Model file for the job. Use its own axes, mm. A direction names the side the tool comes from. Give positions to 0.01 mm unless a question says otherwise; leave off trailing zeros. Loops run counter-clockwise (first coordinate to the right, second up) from the corner with the lowest first, then second, coordinate; pieces in that order, holes last. Notation, with made-up numbers: M 70,2.5 L 86,2.5 A26 cw 86,25.5 Z; hole C -34,65 d11. An arc over 180 degrees is marked long. Answer in a Markdown table with one row per item.
```python
from build123d import *

# Parameters (mm, degrees)
STOCK_ECCENTRIC_START               = 21
STOCK_ECCENTRIC_SHAFT_1_OUTLINE_R   = 10
STOCK_ECCENTRIC_SHAFT_1_OUTLINE_R_2 = 1.5
STOCK_ECCENTRIC_SHAFT_1_DEPTH       = 9
STOCK_ECCENTRIC_START_2             = 30
STOCK_ECCENTRIC_SHAFT_1_2_DEPTH     = 1
BOSS_EXTRUDE1_START                 = 1
SKETCH1_R                           = 10
SKETCH1_R_2                         = 1.5
BOSS_EXTRUDE1_DEPTH                 = 1
CUT_EXTRUDE1_START                  = -1
CUT_EXTRUDE1_DEPTH                  = 1


# Read off the part's stored shape, not the designer's step: Stock-Eccentric Shaft-1
with BuildPart() as part:
    # Stock-Eccentric Shaft-1 outline → Stock-Eccentric Shaft-1 (new body)
    with BuildSketch(Plane(origin=(0, 0, 0), x_dir=(1, 0, 0), z_dir=(0, 1, 0)).offset(STOCK_ECCENTRIC_START)):
        with Locations((-2.5, 0)):
            Circle(STOCK_ECCENTRIC_SHAFT_1_OUTLINE_R)
        with Locations((-4, 0)):
            Circle(STOCK_ECCENTRIC_SHAFT_1_OUTLINE_R_2, mode=Mode.SUBTRACT)
        with Locations((4, 0)):
            Circle(STOCK_ECCENTRIC_SHAFT_1_OUTLINE_R_2, mode=Mode.SUBTRACT)
    extrude(amount=STOCK_ECCENTRIC_SHAFT_1_DEPTH)

    # Stock-Eccentric Shaft-1 2 outline → Stock-Eccentric Shaft-1 2 (add)
    with BuildSketch(Plane(origin=(0, 0, 0), x_dir=(1, 0, 0), z_dir=(0, 1, 0)).offset(STOCK_ECCENTRIC_START_2)):
        with BuildLine():
            ThreePointArc((-10.712142643, 2.5), (-8.817418729, 6.576710953), (-5.45, 9.554972527))
            ThreePointArc((-5.45, 9.554972527), (-9.734494483, 6.903773575), (-12.182458366, 2.5))
            Line((-12.182458366, 2.5), (-10.712142643, 2.5))
        make_face()
        with BuildLine():
            ThreePointArc((-12.182458366, -2.5), (-9.734494483, -6.903773575), (-5.45, -9.554972527))
            ThreePointArc((-5.45, -9.554972527), (-8.817418729, -6.576710953), (-10.712142643, -2.5))
            Line((-10.712142643, -2.5), (-12.182458366, -2.5))
        make_face()
    extrude(amount=STOCK_ECCENTRIC_SHAFT_1_2_DEPTH)

    # Sketch1 → Boss-Extrude1 (add)
    # profile 1 of 4: a face of its own
    with BuildSketch(Plane.XZ.offset(-21).offset(BOSS_EXTRUDE1_START)):
        with BuildLine():
            Line((7.928326807, -3.5), (7.8, -3.5))
            Line((7.8, -3.5), (7.8, 3.5))
            Line((7.8, 3.5), (7.928326807, 3.5))
            ThreePointArc((7.928326807, 3.5), (-13.5, 0), (7.928326807, -3.5))
        make_face()
        with Locations(Location((-2.5, 0, 0), (0, 0, 252.842462628))):
            Circle(SKETCH1_R, mode=Mode.SUBTRACT)
    # profile 2 of 4: a face of its own
    with BuildSketch(Plane.XZ.offset(-21).offset(BOSS_EXTRUDE1_START)):
        with Locations(Location((-2.5, 0, 0), (0, 0, 252.842462628))):
            Circle(SKETCH1_R)
        with Locations(Location((4, 0, 0), (0, 0, 90))):
            Circle(SKETCH1_R_2, mode=Mode.SUBTRACT)
        with Locations(Location((-4, 0, 0), (0, 0, 90))):
            Circle(SKETCH1_R_2, mode=Mode.SUBTRACT)
    # profile 3 of 4: a face of its own
    with BuildSketch(Plane.XZ.offset(-21).offset(BOSS_EXTRUDE1_START)):
        with BuildLine():
            Line((7.8, 3.5), (7.8, -3.5))
            Line((7.8, -3.5), (7.928326807, -3.5))
            ThreePointArc((7.928326807, -3.5), (8.356141001, -1.773189939), (8.5, 0))
            ThreePointArc((8.5, 0), (8.356141001, 1.773189939), (7.928326807, 3.5))
            Line((7.928326807, 3.5), (7.8, 3.5))
        make_face()
    # profile 4 of 4: a face of its own
    with BuildSketch(Plane.XZ.offset(-21).offset(BOSS_EXTRUDE1_START)):
        with BuildLine():
            ThreePointArc((8.5, 0), (8.356141001, -1.773189939), (7.928326807, -3.5))
            Line((7.928326807, -3.5), (10.8, -3.5))
            Line((10.8, -3.5), (10.8, 3.5))
            Line((10.8, 3.5), (7.928326807, 3.5))
            ThreePointArc((7.928326807, 3.5), (8.356141001, 1.773189939), (8.5, 0))
        make_face()
    extrude(amount=-BOSS_EXTRUDE1_DEPTH)

    # Sketch2 → Cut-Extrude1 (cut)
    with BuildSketch(Plane(origin=(0, 31, 0), x_dir=(1, 0, 0), z_dir=(0, 1, 0)).offset(CUT_EXTRUDE1_START)):
        with BuildLine():
            ThreePointArc((-5.45, 9.554972527), (-6.473664245, 9.176600268), (-7.45, 8.688929738))
            Line((-7.45, 8.688929738), (-7.45, 8.093052576))
            ThreePointArc((-7.45, 8.093052576), (-6.491286659, 8.880495342), (-5.45, 9.554972527))
        make_face()
        with BuildLine():
            ThreePointArc((-5.45, -9.554972527), (-6.491286659, -8.880495342), (-7.45, -8.093052576))
            Line((-7.45, -8.093052576), (-7.45, -8.688929738))
            ThreePointArc((-7.45, -8.688929738), (-6.473664245, -9.176600268), (-5.45, -9.554972527))
        make_face()
    extrude(amount=CUT_EXTRUDE1_DEPTH, mode=Mode.SUBTRACT)


solid = part.part
```
Q1. Probe probe 1 along X at (y, z) = (20.65, 0); probe 2 along X at (y, z) = (23.5, 0); probe 3 along Y at (x, z) = (-5.5, -10). List the from-to ranges inside material, lowest first.
Reported:
| item | result |
|---|---|
| probe 1 | -13.5 to -5.5, -2.5 to 2.5, 5.5 to 10.8 |
| probe 2 | -12.5 to -5.5, -2.5 to 2.5, 5.5 to 7.5 |
| probe 3 | 20 to 21 |
Q2. Drop flat-ended pins along their axis: pin 1 (2 mm diameter, centred on x = 5, y = 27.5, fed in from -Z); pin 2 (1.5 mm diameter, centred on x = -10, y = 27, fed in from -Z); pin 3 (0.8 mm diameter, centred on x = -11.5, y = 30.5, fed in from +Z). Give the stop position or say it passes through.
Reported:
| item | result |
|---|---|
| pin 1 | z = -7.6 |
| pin 2 | z = -7.38 |
| pin 3 | z = 5.1 |
Q3. Saw through at A-A (z = 0). Give the cut face in (x, y).
Reported:
| item | result |
|---|---|
| outline | M -13.5,20 L -5.5,20 L -5.5,30 L -12.5,30 L -12.5,21 L -13.5,21 Z; M -2.5,20 L 2.5,20 L 2.5,30 L -2.5,30 Z; M 5.5,20 L 10.8,20 L 10.8,21 L 7.5,21 L 7.5,30 L 5.5,30 Z |
Q4. 3-axis set-ups, long thin cutter, end or side, ignore diameter. For faces 1 (the face through (-11.5, 30.5, -2.5)), 2 (the face through (-9.525, 30.493, -5.502)), 3 (the face through (-2, 20, 0)), 4 (the face through (8, 21, 0)), 5 (the face through (9.4, 20.5, 3.5)): which of +Z, -Z, +X, -X, +Y, -Y reach the whole face in a straight line?
Reported:
| item | result |
|---|---|
| face 1 | +X, -X, +Y |
| face 2 | +X, +Y |
| face 3 | +Z, -Z, +X, -X, -Y |
| face 4 | +Y |
| face 5 | +Z, +X, +Y, -Y |
Q5. Saw through at B-B (x = 3). Give the cut face in (y, z), and give its area (3 significant figures).
Reported:
| item | result |
|---|---|
| outline | M 20,-9.53 L 21,-9.53 L 21,-8.35 L 30,-8.35 L 30,-1.12 L 20,-1.12 Z; M 20,1.12 L 30,1.12 L 30,8.35 L 21,8.35 L 21,9.53 L 20,9.53 Z |
| area | 147 mm² |
Q6. Saw through at D-D (x = 0.5). Give the cut face in (y, z), and give its area (3 significant figures).
Reported:
| item | result |
|---|---|
| outline | M 20,-10.58 L 21,-10.58 L 21,-9.54 L 30,-9.54 L 30,9.54 L 21,9.54 L 21,10.58 L 20,10.58 Z |
| area | 193 mm² |
Q7. Mould opens along Z. For faces 6 (the face through (-9.48, 30.49, 5.58)), 7 (the face through (9.3, 20.5, -3.5)), 8 (the face through (-10, 31, 5)) say: released by +Z, released by -Z, zero draft, split by the parting line, or undercut.
Reported:
| item | result |
|---|---|
| face 6 | undercut |
| face 7 | released by -Z |
| face 8 | zero draft |
Q8. Saw through at C-C (y = 24.5). Give the cut face in (x, z).
Reported:
| item | result |
|---|---|
| outline | C -2.5,0 d20; hole C -4,0 d3; hole C 4,0 d3 |
